from build123d import *

# Parameters (mm, degrees)
SKETCH1_R           = 2.7
SKETCH1_R_2         = 3.875
BOSS_EXTRUDE1_DEPTH = 3.125
FILLET1_R           = 10


with BuildPart() as part:
    # Sketch1 → Boss-Extrude1 (new body)
    with BuildSketch(Plane(origin=(0, 0, 0), x_dir=(1, 0, 0), z_dir=(0, 1, 0))):
        Polygon((0, 25.810224973), (0, 0), (60, -20.189775027), (78, -20.189775027), (78, 45.810224973), (60, 45.810224973), align=None)
        with Locations((70.074055608, -12.033915485)):
            Circle(SKETCH1_R, mode=Mode.SUBTRACT)
        with Locations((10.074055608, 12.966084515)):
            Circle(SKETCH1_R_2, mode=Mode.SUBTRACT)
        with Locations((70.074055608, 37.966084515)):
            Circle(SKETCH1_R, mode=Mode.SUBTRACT)
        with Locations((70.074055608, 12.966084515)):
            Circle(SKETCH1_R, mode=Mode.SUBTRACT)
        with Locations((30.074055608, 12.966084515)):
            Circle(SKETCH1_R, mode=Mode.SUBTRACT)
    extrude(amount=BOSS_EXTRUDE1_DEPTH)

    # Fillet1
    fillet1_edges = [part.edges().sort_by_distance(p)[0] for p in [
        (60, 1.5625, -45.810224973),
        (78, 1.5625, -45.810224973),
        (78, 1.5625, 20.189775027),
        (60, 1.5625, 20.189775027),
        (0, 1.5625, 0),
        (0, 1.5625, -25.810224973),
    ]]
    fillet(fillet1_edges, radius=FILLET1_R)


solid = part.part
Geometry check sheet. Reference: the model listing, model coordinates, mm. Round coordinates to 2 decimals unless told otherwise and drop trailing zeros. Loops run counter-clockwise (first coordinate to the right, second up) from the corner with the lowest first, then second, coordinate; pieces in that order, holes last. Notation, with made-up numbers: (-36.75, 2.25) - (-10.75, 2.25) arc R22 cw to (-10.75, 17.25) - close; hole circle Ø8 at (2, 84). An arc over 180 degrees is marked (long way). Answer as CSV lines item,"result".
(1) Depth check by flat-ended pin: pin 1 Ø1 at (x, y) = (29.5, 2.5) entering from +Z; pin 2 Ø4.5 at (x, z) = (70.07, -12.97) entering from +Y. Enter the tip coordinate at first touch or a pass-through.
Output values:
pin 1,"stops at z = 10.09"
pin 2,"passes through"
(2) Material ranges on line 1 along Z through (x, y) = (71, 0.75); line 2 along X through (y, z) = (2.6, -14.5); line 3 along Z through (x, y) = (70, 2.3), recorded low to high.
Output values:
line 1,"z = -45.35 to -40.5, -35.43 to -15.5, -10.43 to 9.5, 14.57 to 19.73"
line 2,"x = 0 to 6.52, 13.63 to 27.85, 32.3 to 67.85, 72.3 to 78"
line 3,"z = -45.61 to -40.67, -35.27 to -15.67, -10.27 to 9.33, 14.73 to 19.99"
(3) Cross-section at D-D, the plane z = -23.5. Enter the section's corners in (x, y) (3 decimals), and give its area (3 significant figures).
Output values:
outline,"(1.281, 0) - (78, 0) - (78, 3.125) - (1.281, 3.125) - close"
area,"240 mm²"
(4) Cross-section at A-A, the plane z = -14.5. Enter the section's corners in (x, y) (3 decimals).
Output values:
outline,"(0, 0) - (6.516, 0) - (6.516, 3.125) - (0, 3.125) - close; (13.633, 0) - (27.852, 0) - (27.852, 3.125) - (13.633, 3.125) - close; (32.296, 0) - (67.852, 0) - (67.852, 3.125) - (32.296, 3.125) - close; (72.296, 0) - (78, 0) - (78, 3.125) - (72.296, 3.125) - close"
(5) Cross-section at B-B, the plane y = 0.95. Give the number of separate pieces and of enclosed holes in the cut face, and give its area (3 significant figures).
Output values:
separate pieces,"1"
enclosed holes,"5"
area,"3,740 mm²"
(6) Release check for a two-part mould opening along X. For faces 1 (the face through (47, 3.125, -13)), 2 (the face through (13.77, 1.54, -14.13)), 3 (the face through (0, 2, -13)) record: released by +X, released by -X, zero draft, split by the parting line, or undercut.
Output values:
face 1,"zero draft"
face 2,"undercut"
face 3,"released by -X"
(7) Cross-section at C-C, the plane x = 13. Enter the section's corners in (y, z) (3 decimals).
Output values:
outline,"(0, -30.144) - (3.125, -30.144) - (3.125, -15.507) - (0, -15.507) - close; (0, -10.426) - (3.125, -10.426) - (3.125, 4.374) - (0, 4.374) - close"
